```python
from build123d import *

# Parameters (mm, degrees)
ESBO_O1_W                = 37
ESBO_O1_H                = 20
RESSALTO_EXTRUS_O1_DEPTH = 1.5
ESBO_O2_R                = 1
CORTE_EXTRUS_O1_DEPTH    = 2.5
ESBO_O3_R                = 0.5
RESSALTO_EXTRUS_O2_DEPTH = 20
ESBO_O4_W                = 1
ESBO_O4_H                = 8
RESSALTO_EXTRUS_O3_DEPTH = 1
ESBO_O5_R                = 0.707106781
RESSALTO_EXTRUS_O4_DEPTH = 8


with BuildPart() as part:
    # Esboço1 → Ressalto-extrusão1 (new body)
    with BuildSketch(Plane.XY):
        Rectangle(ESBO_O1_W, ESBO_O1_H)
    extrude(amount=RESSALTO_EXTRUS_O1_DEPTH)

    # Esboço2 → Corte-extrusão1 (cut, through all)
    with BuildSketch(Plane.XY.offset(1.5)):
        with Locations((16.5, 8)):
            Circle(ESBO_O2_R)
        with Locations((16.5, -8)):
            Circle(ESBO_O2_R)
    extrude(amount=-CORTE_EXTRUS_O1_DEPTH, mode=Mode.SUBTRACT)

    # Esboço3 → Ressalto-extrusão2 (add)
    with BuildSketch(Plane.XY.offset(1.5)):
        with Locations((-12.5, 4)):
            Circle(ESBO_O3_R)
        with Locations((-4, 4)):
            Circle(ESBO_O3_R)
        with Locations((7, 4)):
            Circle(ESBO_O3_R)
        with Locations((7, -4)):
            Circle(ESBO_O3_R)
        with Locations((-4, -4)):
            Circle(ESBO_O3_R)
        with Locations((-12.5, -4)):
            Circle(ESBO_O3_R)
    extrude(amount=RESSALTO_EXTRUS_O2_DEPTH)

    # Esboço4 → Ressalto-extrusão3 (add)
    with BuildSketch(Plane.XY.offset(21.5)):
        with Locations((-12.5, 0)):
            Rectangle(ESBO_O4_W, ESBO_O4_H)
        with Locations((-4, 0)):
            Rectangle(ESBO_O4_W, ESBO_O4_H)
        with Locations((7, 0)):
            Rectangle(ESBO_O4_W, ESBO_O4_H)
    extrude(amount=RESSALTO_EXTRUS_O3_DEPTH)

    # Esboço5 → Ressalto-extrusão4 (add)
    with BuildSketch(Plane.XZ.offset(4)):
        with Locations((-12.5, 22)):
            Circle(ESBO_O5_R)
        with Locations((-4, 22)):
            Circle(ESBO_O5_R)
        with Locations((7, 22)):
            Circle(ESBO_O5_R)
    extrude(amount=-RESSALTO_EXTRUS_O4_DEPTH)


solid = part.part
```
CAD build for the part. Positions are in the model's coordinates, mm. A direction names the side the tool comes from. Coordinates: 2 decimals unless noted, no trailing zeros. Order: outer loops, then holes, each group sorted by start corner. A loop starts at its lowest first (then second) coordinate and runs counter-clockwise, first axis right, second up. Notation, with made-up numbers: (71, 59) -> (125, 59) arc R16 ccw to (125, 75) -> close; hole circle Ø10 at (71, 56). An arc over 180 degrees is marked (long way). Use one line per item in the form item = value. Start each with the question number.
1) Tool access for faces 1 (the cylindrical face through (-12.6, -0.1, 22.7)), 2 (the flat face through (-4, -4, 22)), 3 (the flat face through (-13, 4, 22)): list every direction of +Z, -Z, +X, -X, +Y, -Y with a clear straight run to the whole face (end or side of a thin tool).
2) Pull direction Y, two halves, no side cores. Call faces 4 (the flat face through (0, 10, 1)), 5 (the cylindrical face through (-4.065, -3.504, 11.36)), 6 (the flat face through (-13, -4, 22)): +Y half, -Y half, draft (parallel to the pull), parting line (faces both ways), or undercut.
3) Band-saw the part on A-A on z = 22. Give the cut face in (x, y), then the cut area to 3 significant figures.
4) Drill centre lines: L1, parallel to Y at x = 16.5, z = 0.8; L2, parallel to Z at x = -8.5, y = 8.25; L3, parallel to Z at x = -13, y = -2. Where is each one in solid material? Low to high. Write a range as [from, to].
5) Band-saw the part on C-C on y = 1.5. Give the cut face in (x, z), then the cut area to 3 significant figures.
6) Band-saw the part on D-D on z = 16. Give the cut face in (x, y), then the cut area to 3 significant figures.
7) Band-saw the part on B-B on x = -4. Give the cut face in (y, z).
8) Drop flat-ended pins along their axis: pin 1 (1.5 mm diameter, centred on y = -4, z = 3, fed in from -X); pin 2 (0.6 mm diameter, centred on x = 7.5, z = 22.5, fed in from +Y); pin 3 (0.6 mm diameter, centred on x = 7, y = 4.5, fed in from +Z). Give the stop position or say it passes through.
Entries:
q1.face_1 = none
q1.face_2 = +Z, +X, -X, -Y
q1.face_3 = +Z, +X, -X, +Y
q2.face_4 = +Y half
q2.face_5 = undercut
q2.face_6 = -Y half
q3.outline = (-13.21, -4) -> (-11.79, -4) -> (-11.79, 4) -> (-13.21, 4) -> close; (-4.71, -4) -> (-3.29, -4) -> (-3.29, 4) -> (-4.71, 4) -> close; (6.29, -4) -> (7.71, -4) -> (7.71, 4) -> (6.29, 4) -> close
q3.area = 33.9 mm2
q4.L1 = [-10, -9], [-7, 7], [9, 10]
q4.L2 = [0, 1.5]
q4.L3 = [0, 1.5], [21.5, 22.5]
q5.outline = (-18.5, 0) -> (18.5, 0) -> (18.5, 1.5) -> (-18.5, 1.5) -> close; circle Ø1.41 at (-12.5, 22); circle Ø1.41 at (-4, 22); circle Ø1.41 at (7, 22)
q5.area = 60.2 mm2
q6.outline = circle Ø1 at (-12.5, -4); circle Ø1 at (-12.5, 4); circle Ø1 at (-4, -4); circle Ø1 at (-4, 4); circle Ø1 at (7, -4); circle Ø1 at (7, 4)
q6.area = 4.71 mm2
q7.outline = (-10, 0) -> (10, 0) -> (10, 1.5) -> (4.5, 1.5) -> (4.5, 21.5) -> (4, 21.5) -> (4, 22.71) -> (-4, 22.71) -> (-4, 21.5) -> (-4.5, 21.5) -> (-4.5, 1.5) -> (-10, 1.5) -> close; hole (-3.5, 1.5) -> (3.5, 1.5) -> (3.5, 21.29) -> (-3.5, 21.29) -> close
q8.pin_1 = -13
q8.pin_2 = 4
q8.pin_3 = 21.5
